```python
from build123d import *

# Parameters (mm, degrees)
F1_DEPTH = 8
F2_W     = 14.5
F2_H     = 12
F2_W_2   = 22.5
F3_DEPTH = 8
F4_R     = 1.6
F5_DEPTH = 32
F6_R     = 1.6
F7_DEPTH = 24
F8_SIZE  = 2
F9_SIZE  = 2


with BuildPart() as f1:
    # F0 (on Top) → F1 (new body)
    with BuildSketch(Plane.XY):
        Polygon((12, 22), (-12, 22), (-12, 12), (-16, 0), (-16, -10), (16, -10), (16, 0), (12, 12), align=None)
    extrude(amount=F1_DEPTH)

    # F2 (on face) → F3 (cut, through all)
    with BuildSketch(Plane.XY.offset(8)):
        with Locations((0, 16)):
            Rectangle(F2_W, F2_H)
        with Locations((0, -4)):
            Rectangle(F2_W_2, F2_H)
    extrude(amount=-F3_DEPTH, mode=Mode.SUBTRACT)

    # F4 (on face) → F5 (cut, through all)
    with BuildSketch(Plane.YZ.offset(16)):
        with Locations((-6, 4)):
            Circle(F4_R)
    extrude(amount=-F5_DEPTH, mode=Mode.SUBTRACT)

    # F6 (on face) → F7 (cut, through all)
    with BuildSketch(Plane.YZ.offset(12)):
        with Locations((18, 4)):
            Circle(F6_R)
    extrude(amount=-F7_DEPTH, mode=Mode.SUBTRACT)

    # F8
    f8_edges = [f1.edges().sort_by_distance(p)[0] for p in [
        (-11.25, 2, 4),
        (11.25, 2, 4),
        (-7.25, 10, 4),
        (7.25, 10, 4),
    ]]
    chamfer(f8_edges, length=F8_SIZE)

    # F9
    f9_edges = [f1.edges().sort_by_distance(p)[0] for p in [
        (-13.625, -10, 8),
        (-13.625, -10, 0),
        (0, 2, 8),
        (0, 2, 0),
        (13.625, -10, 8),
        (13.625, -10, 0),
        (9.625, 22, 8),
        (0, 10, 8),
        (0, 10, 0),
        (-9.625, 22, 8),
        (-9.625, 22, 0),
        (9.625, 22, 0),
    ]]
    chamfer(f9_edges, length=F9_SIZE)


solid = f1.part
```
Can you work these out from the model? Positions are in its coordinate system, mm. A direction names the side the tool comes from. Give positions to 0.01 mm unless a question says otherwise; leave off trailing zeros. Order: outer loops, then holes, each group sorted by start corner. A loop starts at its lowest first (then second) coordinate and runs counter-clockwise, first axis right, second up. Notation, with made-up numbers: (59, 88) - (89, 88) arc R23 ccw to (89, 109) - close; hole circle Ø2 at (59, 85). An arc over 180 degrees is marked (long way). Use a Markdown table: item, result. Add a question column.
Q1. If we section it at C-C on z = 0.75: Write out the boundary of the cut face in (x, y).
Q2. If we mould it in two halves opening along Z, with no side actions, what happens to faces 6 (the flat face through (-14, -9, 1)), 7 (the flat face through (11.25, -4, 4)), 8 (the cylindrical face through (-13.59, -4.52, 3.39))? For each: released by +Z, released by -Z, zero draft, split by the parting line, or undercut.
Q3. If we section it at D-D on x = -1.5: Write out the boundary of the cut face in (y, z).
Q4. If we section it at B-B on x = -13.5: Write out the boundary of the cut face in (y, z), plus the area to 3 significant figures.
Q5. Please list where these lines run through material, in increasing order: line 1 along X through (y, z) = (12, 1.25); line 2 along Z through (x, y) = (13.8, -6).
Q6. On a 3-axis mill with a long thin cutter (end or side, diameter ignored), from which of +Z, -Z, +X, -X, +Y, -Y can I reach the whole of each face in a straight line? I mean faces 1 (the flat face through (10.11, 1.14, 4.06)), 2 (the flat face through (0, 9, 7)), 3 (the flat face through (16, -4, 4)), 4 (the flat face through (0, 2, 4)), 5 (the flat face through (-6.11, 10.86, 4.06)). Say none if no direction works.
Q7. I'm going to push flat-ended pins straight in: pin 1 (3 mm diameter, centred on y = 18, z = 4, fed in from +X); pin 2 (3 mm diameter, centred on x = -1, z = 5, fed in from +Y); pin 3 (4 mm diameter, centred on x = 3.5, z = 4.5, fed in from +Y); pin 4 (2 mm diameter, centred on x = 2.5, z = 5, fed in from -Y). Where does each tip first touch, or does it pass through?
Q8. If we section it at A-A on y = -4: Write out the boundary of the cut face in (x, z).
Answers follow:
| question | item | result |
|---|---|---|
| 1 | outline | (-16, -8.75) - (-11.25, -8.75) - (-11.25, 0) - (-8, 3.25) - (8, 3.25) - (11.25, 0) - (11.25, -8.75) - (16, -8.75) - (16, 0) - (12, 12) - (12, 20.75) - (7.25, 20.75) - (7.25, 12) - (4, 8.75) - (-4, 8.75) - (-7.25, 12) - (-7.25, 20.75) - (-12, 20.75) - (-12, 12) - (-16, 0) - close |
| 2 | face 6 | released by -Z |
| 2 | face 7 | zero draft |
| 2 | face 8 | undercut |
| 3 | outline | (2, 2) - (4, 0) - (8, 0) - (10, 2) - (10, 6) - (8, 8) - (4, 8) - (2, 6) - close |
| 4 | outline | (-10, 2) - (-8, 0) - (7.5, 0) - (7.5, 8) - (-8, 8) - (-10, 6) - close; hole circle Ø3.2 at (-6, 4) |
| 4 | area | 128 mm^2 |
| 5 | line 1 | x = -12 to -7.25, 7.25 to 12 |
| 5 | line 2 | z = 0 to 2.4, 5.6 to 8 |
| 6 | face 1 | -Y |
| 6 | face 2 | +Z, +Y |
| 6 | face 3 | +Z, -Z, +X, +Y, -Y |
| 6 | face 4 | +Z, -Z, -Y |
| 6 | face 5 | +Y |
| 7 | pin 1 | passes through |
| 7 | pin 2 | stops at y = 10 |
| 7 | pin 3 | stops at y = 10.25 |
| 7 | pin 4 | stops at y = 2 |
| 8 | outline | (-16, 0) - (-11.25, 0) - (-11.25, 8) - (-16, 8) - close; (11.25, 0) - (16, 0) - (16, 8) - (11.25, 8) - close |
